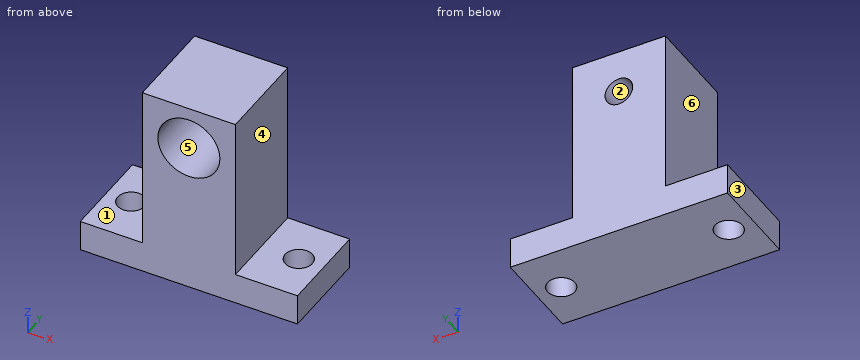
from build123d import *

# Parameters (mm, degrees)
F1_DEPTH       = 30
F3_D           = 8.9
F3_CBORE_D     = 20
F3_CBORE_DEPTH = 20
F5_D           = 8.8


with BuildPart() as f1:
    # F0 (on Front) → F1 (new body)
    with BuildSketch(Plane.XZ):
        Polygon((0, 10), (0, 0), (70, 0), (70, 10), (50, 10), (50, 63.1707229285), (20, 63.1707229285), (20, 10), align=None)
    extrude(amount=F1_DEPTH)

    # F3 (through all)
    with Locations(Plane.XZ.offset(30)):
        with Locations((35, 49.1707229285)):
            CounterBoreHole(F3_D / 2, F3_CBORE_D / 2, F3_CBORE_DEPTH)

    # F5 (through all)
    with Locations(Plane(origin=(0, 0, 0), x_dir=(1, 0, 0), z_dir=(0, 0, -1))):
        with Locations((8, 15), (62, 15)):
            Hole(F5_D / 2)


solid = f1.part
The model under review builds one solid part; all positions refer to its coordinate system, in mm. Face numbers are marked on the shaded views. A direction names the side the tool comes from. Give positions to 0.01 mm unless a question says otherwise; leave off trailing zeros. Write each loop counter-clockwise with the first axis right and the second up, starting at its lowest first coordinate (ties: lowest second). Pieces come first, ordered by that corner, then holes. Notation, with made-up numbers: M 12.5,-37 L 51.5,-37 A22 cw 51.5,-1 Z; hole C -26,52.5 d11. An arc over 180 degrees is marked long. One line per question, with ' | ' between items. Start each with the question number.
Item 1: Draft analysis for pull direction Z (two halves, no side actions). For the marked faces 1, 2 and 3, state which applies: released by +Z, released by -Z, zero draft, split by the parting line, or undercut.
Item 2: Wall thickness on line 1 (X direction, y = -14.25, z = 49); line 2 (Z direction, x = 35, y = -2); line 3 (Z direction, x = 54.5, y = -2.25): over which ranges is each line inside the solid? List them lowest first. Write a range as from..to.
Item 3: For pin 1 (6 mm diameter, centred on x = 13, y = -10, fed in from +Z); pin 2 (2 mm diameter, centred on x = 17.5, z = 50, fed in from +Y); pin 3 (4 mm diameter, centred on y = -3.5, z = 55, fed in from -X); pin 4 (10 mm diameter, centred on x = 35.5, z = 48.5, fed in from -Y), all flat-tipped, find the tip position at first contact; note any pin that passes through.
Item 4: We need section B-B on x = 62. Write out the cut boundary in (y, z), plus the area to 3 significant figures.
Item 5: We need section D-D on y = -1.75. Write out the cut boundary in (x, z), plus the area to 3 significant figures.
Item 6: We need section A-A on y = -15. Write out the cut boundary in (x, z), plus the area to 3 significant figures.
Item 7: We need section C-C on z = 37. Write out the cut boundary in (x, y), plus the area to 3 significant figures.
Item 8: For the marked faces 4, 5 and 6, list the 3-axis set-ups (+Z, -Z, +X, -X, +Y, -Y) from which the entire face can be reached by the end or side of a thin tool; tool diameter is ignored.
Results found:
1) face 1: released by +Z | face 2: undercut | face 3: zero draft
2) line 1: x = 20..25, 45..50 | line 2: z = 0..44.72, 53.62..63.17 | line 3: z = 0..10
3) pin 1: stops at z = 10 | pin 2: passes through | pin 3: stops at x = 20 | pin 4: stops at y = -10
4) outline: M -30,0 L -19.4,0 L -19.4,10 L -30,10 Z; M -10.6,0 L 0,0 L 0,10 L -10.6,10 Z | area: 212 mm2
5) outline: M 0,0 L 70,0 L 70,10 L 50,10 L 50,63.17 L 20,63.17 L 20,10 L 0,10 Z; hole C 35,49.17 d8.9 | area: 2,230 mm2
6) outline: M 0,0 L 3.6,0 L 3.6,10 L 0,10 Z; M 12.4,0 L 57.6,0 L 57.6,10 L 50,10 L 50,63.17 L 20,63.17 L 20,10 L 12.4,10 Z; M 66.4,0 L 70,0 L 70,10 L 66.4,10 Z; hole C 35,49.17 d20 | area: 1,800 mm2
7) outline: M 20,-30 L 50,-30 L 50,0 L 20,0 Z | area: 900 mm2
8) face 4: +Z, +X, +Y, -Y | face 5: -Y | face 6: +Z, -X, +Y, -Y
